Can you work these out from the drawing? Everything is in mm from the part's minimum corner. Give positions to 0.01 mm unless a question says otherwise; leave off trailing zeros. Order: outer loops, then holes, each group sorted by start corner. A loop starts at its lowest first (then second) coordinate and runs counter-clockwise, first axis right, second up. Notation, with made-up numbers: M 42,5.5 L 70,5.5 A7 cw 70,11.5 Z; hole C 37.25,27.5 d8. An arc over 180 degrees is marked long. Answer as a JSON object with one key per item and string values.
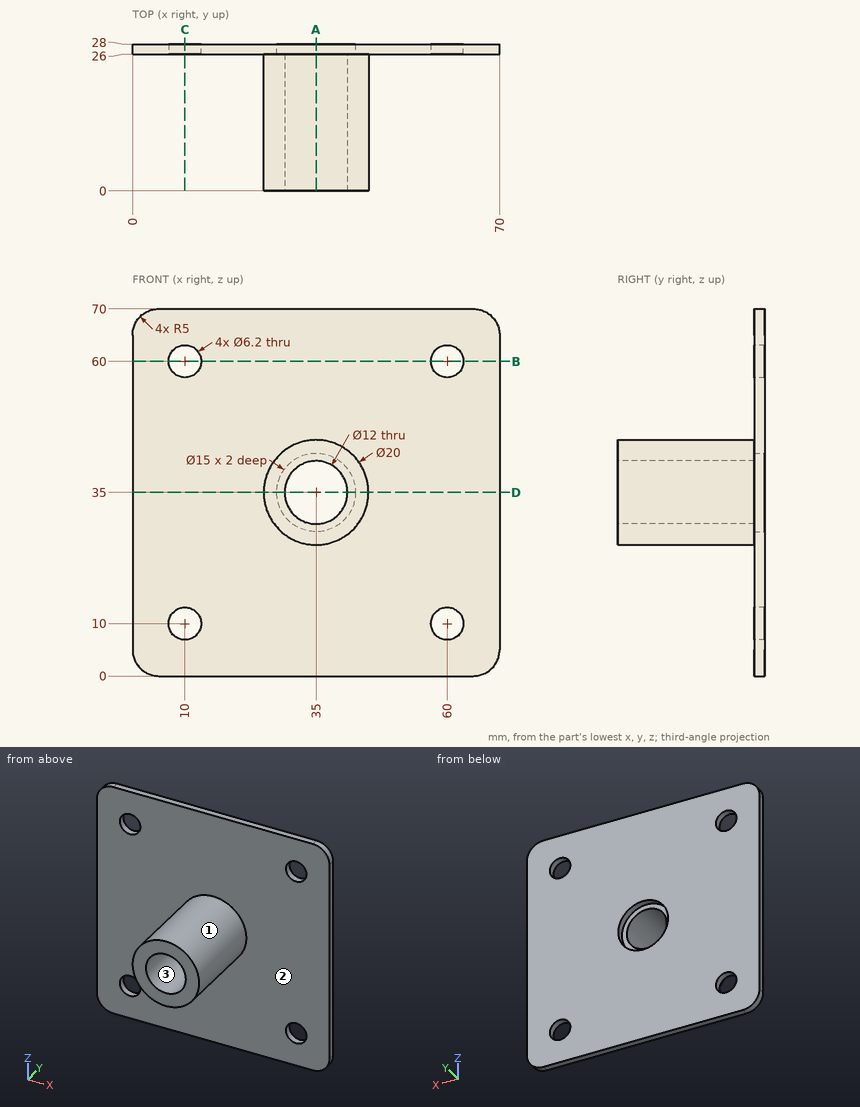
1) I need wall thicknesses on L1, parallel to X at y = 27, z = 60; L2, parallel to X at y = 26.5, z = 35. Which ranges of each line are inside material? Lowest first, please.
Results found:
{"L1": "x = 0 to 6.9, 13.1 to 56.9, 63.1 to 70", "L2": "x = 0 to 27.5, 42.5 to 70"}
2) I want a section at B-B on z = 60. Write out the boundary of the cut face in (x, y), and give its area (3 significant figures).
Results found:
{"outline": "M 0,26 L 6.9,26 L 6.9,28 L 0,28 Z; M 13.1,26 L 56.9,26 L 56.9,28 L 13.1,28 Z; M 63.1,26 L 70,26 L 70,28 L 63.1,28 Z", "area": "115 mm²"}
3) I'm going to push flat-ended pins straight in: pin 1 Ø1.5 at (x, y) = (36, 12) entering from +Z; pin 2 Ø19.5 at (x, z) = (35, 35) entering from -Y; pin 3 Ø2 at (x, z) = (24, 55) entering from -Y; pin 4 Ø10 at (y, z) = (4, 30) entering from +X. Where does each tip first touch, or does it pass through?
Results found:
{"pin 1": "stops at z = 45", "pin 2": "stops at y = 0", "pin 3": "stops at y = 26", "pin 4": "stops at x = 45"}
4) I want a section at D-D on z = 35. Write out the boundary of the cut face in (x, y), and give its area (3 significant figures).
Results found:
{"outline": "M 0,26 L 25,26 L 25,0 L 29,0 L 29,26 L 27.5,26 L 27.5,28 L 0,28 Z; M 41,0 L 45,0 L 45,26 L 70,26 L 70,28 L 42.5,28 L 42.5,26 L 41,26 Z", "area": "318 mm²"}
5) Thinking about a two-plate mould opening in Z: for the marked faces 1, 2 and 3, which applies, pulls with the +Z half, pulls with the -Z half, needs draft (parallel to the pull), parting line crosses it, or undercut?
Results found:
{"face 1": "parting line crosses it", "face 2": "needs draft", "face 3": "undercut"}
6) I want a section at C-C on x = 10. Write out the boundary of the cut face in (y, z), and give its area (3 significant figures).
Results found:
{"outline": "M 26,0 L 28,0 L 28,6.9 L 26,6.9 Z; M 26,13.1 L 28,13.1 L 28,56.9 L 26,56.9 Z; M 26,63.1 L 28,63.1 L 28,70 L 26,70 Z", "area": "115 mm²"}
7) I want a section at A-A on x = 35. Write out the boundary of the cut face in (y, z).
Results found:
{"outline": "M 0,25 L 26,25 L 26,0 L 28,0 L 28,27.5 L 26,27.5 L 26,29 L 0,29 Z; M 0,41 L 26,41 L 26,42.5 L 28,42.5 L 28,70 L 26,70 L 26,45 L 0,45 Z"}
